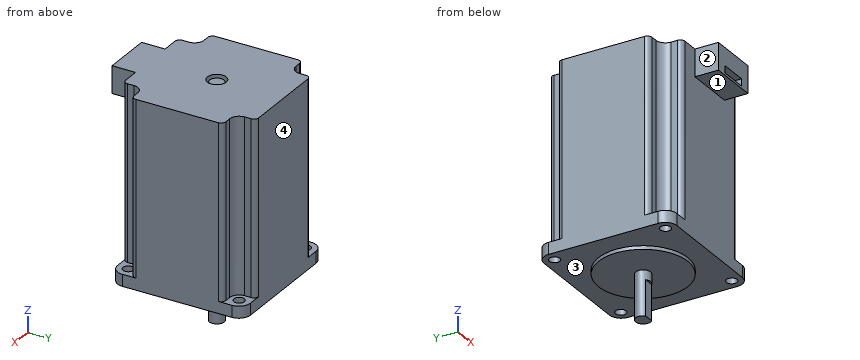
```python
from build123d import *

# Parameters (mm, degrees)
SKETCH_1_W          = 56.5
SKETCH_1_H          = 56.5
EXTRUDE_1_DEPTH     = 79
FILLET_1_R          = 5
SKETCH_2_W          = 27.937414654
SKETCH_2_H          = 17.525111135
CUT_EXTRUDE_1_DEPTH = 74
FILLET_2_R          = 4
FILLET_3_R          = 2
SKETCH_3_R          = 19
EXTRUDE_2_DEPTH     = 1.5
SKETCH_4_R          = 4
CUT_EXTRUDE_2_DEPTH = 3
SKETCH_5_R          = 3
EXTRUDE_3_DEPTH     = 2
SKETCH_6_R          = 3.175
EXTRUDE_4_DEPTH     = 19
SKETCH_7_R          = 2.25
CUT_EXTRUDE_3_DEPTH = 21
SKETCH_8_W          = 21
SKETCH_8_H          = 11.5
EXTRUDE_5_DEPTH     = 10
SKETCH_9_W          = 12
SKETCH_9_H          = 3
CUT_EXTRUDE_4_DEPTH = 5
SKETCH_10_W         = 15
SKETCH_10_H         = 3.472611371
CUT_EXTRUDE_6_DEPTH = 113.36325022


with BuildPart() as part:
    # 草图1 → 凸台-拉伸1 (new body)
    with BuildSketch(Plane.XY):
        with Locations((28.25, 28.25)):
            Rectangle(SKETCH_1_W, SKETCH_1_H)
    extrude(amount=EXTRUDE_1_DEPTH)

    # 圆角1
    fillet_1_edges = [part.edges().sort_by_distance(p)[0] for p in [
        (0, 56.5, 39.5),
        (56.5, 56.5, 39.5),
        (56.5, 0, 39.5),
        (0, 0, 39.5),
    ]]
    fillet(fillet_1_edges, radius=FILLET_1_R)

    # 草图2 → 切除-拉伸1 (cut)
    with BuildSketch(Plane.XY.offset(79)):
        with Locations((-5.218707327, 56.512555568)):
            Rectangle(SKETCH_2_W, SKETCH_2_H)
        with Locations((61.718707327, 56.512555568)):
            Rectangle(SKETCH_2_W, SKETCH_2_H)
        with Locations((61.718707327, -0.012555568)):
            Rectangle(SKETCH_2_W, SKETCH_2_H)
        with Locations((-5.218707327, -0.012555568)):
            Rectangle(SKETCH_2_W, SKETCH_2_H)
    extrude(amount=-CUT_EXTRUDE_1_DEPTH, mode=Mode.SUBTRACT)

    # 圆角2
    fillet_2_edges = [part.edges().sort_by_distance(p)[0] for p in [
        (8.75, 47.75, 42),
        (47.75, 47.75, 42),
        (47.75, 8.75, 42),
        (8.75, 8.75, 42),
    ]]
    fillet(fillet_2_edges, radius=FILLET_2_R)

    # 圆角3
    fillet_3_edges = [part.edges().sort_by_distance(p)[0] for p in [
        (8.75, 56.5, 42),
        (0, 47.75, 42),
        (56.5, 47.75, 42),
        (47.75, 56.5, 42),
        (47.75, 0, 42),
        (56.5, 8.75, 42),
        (0, 8.75, 42),
        (8.75, 0, 42),
    ]]
    fillet(fillet_3_edges, radius=FILLET_3_R)

    # 草图3 → 凸台-拉伸2 (add)
    with BuildSketch(Plane(origin=(0, 0, 0), x_dir=(-1, 0, 0), z_dir=(0, 0, -1))):
        with Locations((-28.25, 28.25)):
            Circle(SKETCH_3_R)
    extrude(amount=EXTRUDE_2_DEPTH)

    # 草图4 → 切除-拉伸2 (cut)
    with BuildSketch(Plane.XY.offset(79)):
        with Locations((28.25, 28.25)):
            Circle(SKETCH_4_R)
    extrude(amount=-CUT_EXTRUDE_2_DEPTH, mode=Mode.SUBTRACT)

    # 草图5 → 凸台-拉伸3 (add)
    with BuildSketch(Plane.XY.offset(76)):
        with Locations((28.25, 28.25)):
            Circle(SKETCH_5_R)
    extrude(amount=EXTRUDE_3_DEPTH)

    # 草图6 → 凸台-拉伸4 (add)
    with BuildSketch(Plane(origin=(0, 0, -1.5), x_dir=(-1, 0, 0), z_dir=(0, 0, -1))):
        with Locations((-28.25, 28.25)):
            Circle(SKETCH_6_R)
    extrude(amount=EXTRUDE_4_DEPTH)

    # 草图7 → 切除-拉伸3 (cut)
    with BuildSketch(Plane(origin=(0, 0, 0), x_dir=(-1, 0, 0), z_dir=(0, 0, -1))):
        with Locations((-51.8, 4.7)):
            Circle(SKETCH_7_R)
        with Locations((-4.7, 4.7)):
            Circle(SKETCH_7_R)
        with Locations((-4.7, 51.8)):
            Circle(SKETCH_7_R)
        with Locations((-51.8, 51.8)):
            Circle(SKETCH_7_R)
    extrude(amount=-CUT_EXTRUDE_3_DEPTH, mode=Mode.SUBTRACT)

    # 草图8 → 凸台-拉伸5 (add)
    with BuildSketch(Plane.XZ):
        with Locations((28.25, 73.25)):
            Rectangle(SKETCH_8_W, SKETCH_8_H)
    extrude(amount=EXTRUDE_5_DEPTH)

    # 草图9 → 切除-拉伸4 (cut)
    with BuildSketch(Plane.XZ.offset(10)):
        with Locations((28.25, 70)):
            Rectangle(SKETCH_9_W, SKETCH_9_H)
    extrude(amount=-CUT_EXTRUDE_4_DEPTH, mode=Mode.SUBTRACT)

    # 草图10 → 切除-拉伸6 (cut, through all)
    with BuildSketch(Plane(origin=(0, 0, 0), x_dir=(0, 0, -1), z_dir=(1, 0, 0))):
        with Locations((13, 24.188694315)):
            Rectangle(SKETCH_10_W, SKETCH_10_H)
    extrude(amount=CUT_EXTRUDE_6_DEPTH, mode=Mode.SUBTRACT)


solid = part.part
```
Source: CAD feature listing. Evaluate the final solid. Frame: model axes, mm. Face numbers are marked on the shaded views. A direction names the side the tool comes from. Round coordinates to 2 decimals unless told otherwise and drop trailing zeros. Order: outer loops, then holes, each group sorted by start corner. A loop starts at its lowest first (then second) coordinate and runs counter-clockwise, first axis right, second up. Notation, with made-up numbers: (-9.75, -17) -> (15.25, -17) arc R26 ccw to (15.25, 14) -> close; hole circle Ø9 at (-38.75, 6). An arc over 180 degrees is marked (long way). Use CSV: the item, a comma, the result in double quotes.
(1) First-contact query: pin 1 Ø10 at (x, z) = (39, 12) entering from -Y; pin 2 Ø5 at (x, y) = (4.7, 4.7) entering from -Z; pin 3 Ø3 at (x, z) = (50.5, 55) entering from +Y; pin 4 Ø12 at (x, y) = (49.5, 5) entering from +Z. Flat tips, straight axial feed; report the tip coordinate or a pass-through.
Report:
pin 1,"y = 0"
pin 2,"z = 0"
pin 3,"y = 48.85"
pin 4,"z = 79"
(2) Section C-C on y = 29.5. Return the cut outline in (x, z).
Report:
outline,"(0, 0) -> (9.29, 0) -> (9.29, -1.5) -> (25.33, -1.5) -> (25.33, -20.5) -> (31.17, -20.5) -> (31.17, -1.5) -> (47.21, -1.5) -> (47.21, 0) -> (56.5, 0) -> (56.5, 79) -> (32.05, 79) -> (32.05, 76) -> (30.98, 76) -> (30.98, 78) -> (25.52, 78) -> (25.52, 76) -> (24.45, 76) -> (24.45, 79) -> (0, 79) -> close"
(3) Section A-A on x = 28.25. Return the cut outline in (y, z) (3 decimals).
Report:
outline,"(-10, 67.5) -> (0, 67.5) -> (0, 0) -> (9.25, 0) -> (9.25, -1.5) -> (25.075, -1.5) -> (25.075, -5.5) -> (25.925, -5.5) -> (25.925, -20.5) -> (31.425, -20.5) -> (31.425, -1.5) -> (47.25, -1.5) -> (47.25, 0) -> (56.5, 0) -> (56.5, 79) -> (32.25, 79) -> (32.25, 76) -> (31.25, 76) -> (31.25, 78) -> (25.25, 78) -> (25.25, 76) -> (24.25, 76) -> (24.25, 79) -> (-10, 79) -> (-10, 71.5) -> (-5, 71.5) -> (-5, 68.5) -> (-10, 68.5) -> close"
(4) Ray query, L1, parallel to Y at x = 51.8, z = 3.1; L2, parallel to Y at x = 28.25, z = 77.45; L3, parallel to Z at x = 47, y = 53.5. Return the intervals inside material, ascending.
Report:
L1,"0.01 to 2.45, 6.95 to 49.55, 54.05 to 56.49"
L2,"-10 to 24.25, 25.25 to 31.25, 32.25 to 56.5"
L3,"0 to 79"
(5) Section D-D on z = 45. Return the cut outline in (x, y).
Report:
outline,"(0, 10.75) arc R2 ccw to (2, 8.75) -> (4.75, 8.75) arc R4 cw to (8.75, 4.75) -> (8.75, 2) arc R2 ccw to (10.75, 0) -> (45.75, 0) arc R2 ccw to (47.75, 2) -> (47.75, 4.75) arc R4 cw to (51.75, 8.75) -> (54.5, 8.75) arc R2 ccw to (56.5, 10.75) -> (56.5, 45.75) arc R2 ccw to (54.5, 47.75) -> (51.75, 47.75) arc R4 cw to (47.75, 51.75) -> (47.75, 54.5) arc R2 ccw to (45.75, 56.5) -> (10.75, 56.5) arc R2 ccw to (8.75, 54.5) -> (8.75, 51.75) arc R4 cw to (4.75, 47.75) -> (2, 47.75) arc R2 ccw to (0, 45.75) -> close"
(6) Access query for the marked faces 1, 2, 3 and 4. Directions: +Z, -Z, +X, -X, +Y, -Y. A direction counts if a zero-diameter tool reaches every point of the face in a straight line with its end or side. Return the directions, or none.
Report:
face 1,"-Z, +X, -X, -Y"
face 2,"+Z, -Z, -X, -Y"
face 3,"-Z"
face 4,"+Z, -Z, +X, -X, +Y"
